Input: part model. Units: mm. Frame: model coordinates. Face numbers are marked on the shaded views. A direction names the side the tool comes from. Give positions to 0.01 mm unless a question says otherwise; leave off trailing zeros. Loops run counter-clockwise (first coordinate to the right, second up) from the corner with the lowest first, then second, coordinate; pieces in that order, holes last. Notation, with made-up numbers: (-17, 41.25) -> (-4, 41.25) arc R30 ccw to (-4, 72.25) -> close; hole circle Ø2 at (16.25, 57). An arc over 180 degrees is marked (long way). Answer as a JSON object with one key per item and string values.
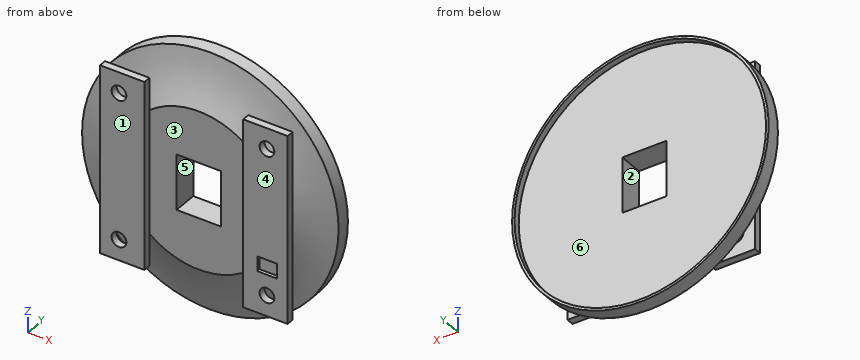
```python
from build123d import *

# Parameters (mm, degrees)
SKETCH7_R             = 25.5
SKETCH7_W             = 9
SKETCH7_H             = 11.2
LENS_SPACER_DEPTH     = 5
SKETCH5_W             = 9
SKETCH5_H             = 38
SKETCH5_R             = 1.5
ATTACHMENT_LEGS_DEPTH = 1.5
LENS_START            = -5
SKETCH8_R             = 26
SKETCH8_R_2           = 25.5
LENS_POSITIONER_DEPTH = 6.25
SKETCH11_W            = 4
SKETCH11_H            = 3
NODE_HOLE_DEPTH       = 0.7


with BuildPart() as part:
    # Sketch7 → Lens Spacer (new body)
    with BuildSketch(Plane.XZ):
        Circle(SKETCH7_R)
        Rectangle(SKETCH7_W, SKETCH7_H, mode=Mode.SUBTRACT)
    extrude(amount=LENS_SPACER_DEPTH)

    # Sketch5 → Attachment Legs (add)
    with BuildSketch(Plane(origin=(0, -5, 0), x_dir=(-1, 0, 0), z_dir=(0, -1, 0))):
        with Locations((-14.525, 0)):
            Rectangle(SKETCH5_W, SKETCH5_H)
        with Locations((-14.825, 14.8)):
            Circle(SKETCH5_R, mode=Mode.SUBTRACT)
        with Locations((-14.825, -14.8)):
            Circle(SKETCH5_R, mode=Mode.SUBTRACT)
        with Locations((14.525, 0)):
            Rectangle(SKETCH5_W, SKETCH5_H)
        with Locations((15.175, -14.8)):
            Circle(SKETCH5_R, mode=Mode.SUBTRACT)
        with Locations((15.175, 14.8)):
            Circle(SKETCH5_R, mode=Mode.SUBTRACT)
    extrude(amount=ATTACHMENT_LEGS_DEPTH)

    # Sketch8 → Lens Positioner (add)
    with BuildSketch(Plane(origin=(0, 0, 0), x_dir=(1, 0, 0), z_dir=(0, 1, 0)).offset(LENS_START)):
        Circle(SKETCH8_R)
        Circle(SKETCH8_R_2, mode=Mode.SUBTRACT)
    extrude(amount=LENS_POSITIONER_DEPTH)

    # Sketch11 → Node Hole (cut)
    with BuildSketch(Plane.XZ.offset(6.5)):
        with Locations((14.868591599, -9.123908481)):
            Rectangle(SKETCH11_W, SKETCH11_H)
    extrude(amount=-NODE_HOLE_DEPTH, mode=Mode.SUBTRACT)

    # Sketch13 → Cut-Revolve1 (revolve, cut)
    with BuildSketch(Plane.XY):
        with BuildLine():
            ThreePointArc((-16, -5), (-20.846735107, -2.830753933), (-26, -1.55))
            Line((-26, -1.55), (-26, -5))
            Line((-26, -5), (-16, -5))
        make_face()
        with BuildLine():
            Line((-23.315412737, -5), (-16, -5))
            ThreePointArc((-16, -5), (-19.657706368, -4.047609039), (-23.315412737, -5))
        make_face()
    revolve(axis=Axis((0, -78.539105243, 0), (0, 1, 0)), mode=Mode.SUBTRACT)


solid = part.part
```
Q1. Pin query (flat end, axial travel): pin 1 (2 mm diameter, centred on x = 9, z = -20, fed in from -Y); pin 2 (3.5 mm diameter, centred on x = -15.175, z = 14.8, fed in from +Y); pin 3 (1.5 mm diameter, centred on y = -4.5, z = 16.5, fed in from +X) (3 decimals); pin 4 (12 mm diameter, centred on x = 9.5, z = 11.5, fed in from -Y). Return the tip coordinate at first contact, or that it passes through.
Evaluation:
{"pin 1": "stops at y = -2.8", "pin 2": "stops at y = 0", "pin 3": "stops at x = 19.025", "pin 4": "stops at y = -6.5"}
Q2. Draft query along Z for the marked faces 1 and 2. Return one class per face: +Z half, -Z half, draft (parallel to the pull), parting line (faces both ways), or undercut.
Evaluation:
{"face 1": "draft", "face 2": "undercut"}
Q3. Section B-B, the plane x = 0. Return the cut outline in (y, z), then the cut area to 3 significant figures.
Evaluation:
{"outline": "(-5, -16) arc R30 cw to (-1.55, -26) -> (1.25, -26) -> (1.25, -25.5) -> (0, -25.5) -> (0, -5.6) -> (-5, -5.6) -> close; (-5, 5.6) -> (0, 5.6) -> (0, 25.5) -> (1.25, 25.5) -> (1.25, 26) -> (-1.55, 26) arc R30 cw to (-5, 16) -> close", "area": "164 mm2"}
Q4. Section D-D, the plane z = -14.8. Give the number of separate pieces and of enclosed holes in the cut face, then the cut area to 3 significant figures.
Evaluation:
{"separate pieces": "5", "enclosed holes": "0", "area": "176 mm2"}
Q5. Ray query, line 1 along X through (y, z) = (-5.55, 14.8) (3 decimals); line 2 along Z through (x, y) = (0, 0.8); line 3 along Z through (x, y) = (-12, -6). Return the intervals inside material, ascending.
Evaluation:
{"line 1": "x = -19.025 to -16.675, -13.675 to -10.025, 10.025 to 13.325, 16.325 to 19.025", "line 2": "z = -26 to -25.5, 25.5 to 26", "line 3": "z = -19 to 19"}
Q6. Section C-C, the plane y = -0.75. Return the cut outline in (x, z), then the cut area to 3 significant figures.
Evaluation:
{"outline": "circle Ø52 at (0, 0); hole (-4.5, -5.6) -> (4.5, -5.6) -> (4.5, 5.6) -> (-4.5, 5.6) -> close", "area": "2,020 mm2"}
Q7. Access query for the marked faces 3, 4, 5 and 6. Directions: +Z, -Z, +X, -X, +Y, -Y. A direction counts if a zero-diameter tool reaches every point of the face in a straight line with its end or side. Return the directions, or none.
Evaluation:
{"face 3": "+Z, -Z, -Y", "face 4": "+Z, -Z, +X, -X, -Y", "face 5": "+Y, -Y", "face 6": "+Y"}
Q8. Section A-A, the plane z = 0. Return the cut outline in (x, y) (3 decimals).
Evaluation:
{"outline": "(-26, -1.55) arc R30 cw to (-16, -5) -> (-19.025, -5) -> (-19.025, -6.5) -> (-10.025, -6.5) -> (-10.025, -5) -> (-4.5, -5) -> (-4.5, 0) -> (-25.5, 0) -> (-25.5, 1.25) -> (-26, 1.25) -> close; (4.5, -5) -> (10.025, -5) -> (10.025, -6.5) -> (19.025, -6.5) -> (19.025, -5) -> (16, -5) arc R30 cw to (26, -1.55) -> (26, 1.25) -> (25.5, 1.25) -> (25.5, 0) -> (4.5, 0) -> close"}
